Autodesk Fusion 360 part; units mm, degrees
sketch "Sketch2" plane through (0, 0, 0) normal (0, 1, 0) x (1, 0, 0)
  line L0 (0, 0) -> (42.015, 0)
  line L1 (42.015, 0) -> (42.015, -15.89)
  line L2 (42.015, -15.89) -> (0, -15.89)
  line L3 (0, -15.89) -> (0, 0)
  circle A0 centre (45.515, -7.945) radius 1.5
  line L4 (42.015, -7.945) -> (48.69, -7.945)
  spline S0 degree 5 poles (42.015, -12.945) (42.5156, -12.7419) (43.4745, -12.3366) (44.7863, -11.7309) (46.2763, -10.9278) (47.6689, -9.93) (48.5399, -8.9364) (48.8392, -7.945) (48.5399, -6.9536) (47.6689, -5.96) (46.2763, -4.9622) (44.7863, -4.1591) (43.4745, -3.5534) (42.5156, -3.1481) (42.015, -2.945) knots 0 0 0 0 0 0 0.1 0.2 0.3 0.4 0.5 0.6 0.7 0.8 0.9 1 1 1 1 1 1
  line L5 (20.92, -15.89) -> (20.92, 0)
  spline S1 degree 5 poles (-0.175, -12.945) (-0.6756, -12.7419) (-1.6345, -12.3366) (-2.9463, -11.7309) (-4.4363, -10.9278) (-5.8289, -9.93) (-6.6999, -8.9364) (-6.9992, -7.945) (-6.6999, -6.9536) (-5.8289, -5.96) (-4.4363, -4.9622) (-2.9463, -4.1591) (-1.6345, -3.5534) (-0.6756, -3.1481) (-0.175, -2.945) knots 0 0 0 0 0 0 0.1 0.2 0.3 0.4 0.5 0.6 0.7 0.8 0.9 1 1 1 1 1 1
  line L6 (40.2192, -13.6735) -> (43.8108, -12.2165)
  line L7 (43.8108, -3.6735) -> (40.2192, -2.2165)
  line L8 (1.6208, -13.6735) -> (-1.9708, -12.2165)
  line L9 (-1.9708, -3.6735) -> (1.6208, -2.2165)
  circle A1 centre (-3.675, -7.945) radius 1.5
  line L10 (-0.175, -7.945) -> (-6.85, -7.945)
  circle A2 centre (20.92, -9.45) radius 1
  circle A3 centre (20.92, -6.45) radius 1
  line L11 (-0.175, -12.945) -> (0, -13.016)
  line L12 (-0.175, -7.945) -> (0, -7.945)
  line L13 (-0.175, -2.945) -> (0, -2.874)
  dimension "d2" = 15.89
  dimension "d3" = 3
  dimension "d5" = 3.5
  dimension "d6" = 10
  dimension "d7" = 2.945
  dimension "d8" = 15.89
  dimension "d19" = 2
  dimension "d20" = 2
  dimension "d21" = 3
  dimension "d22" = 6.45
  dimension "d25" = 49.19
  dimension "d26" = 42.19
  dimension "d27" = 55.54
  dimension "d29" = 7.945
extrude "Extrude1" add sketch "Sketch2" along normal blind 6.35 contours L0 L2 L3 L5 A2 A3 | L0 L1 L2 L5 A2 A3 | L3 S1 L9 A1 L10 L12 L13 | L5 A3 | L5 A3 | L3 S1 L8 A1 L10 L11 L12 | L1 A0 L4 S0 | L1 A0 L4 S0 | L5 A2 | L5 A2
extrude "Extrude2" add sketch "Sketch2" against normal blind 3.56 contours L0 L2 L3 L5 A2 A3 | L0 L1 L2 L5 A2 A3 | L5 A3 | L5 A3 | L5 A2 | L5 A2
extrude "Extrude3" cut sketch "Sketch2" against normal blind 25 contours L5 A3 | L5 A3 | L5 A2 | L5 A2
equation "d5 = d4 - 1.5 mm - d3 / 2"
equation "d7 = ( d8 - d6 ) / 2"
equation "d12 = -9.91 mm + 6.35 mm"
equation "d29 = d2 / 2"
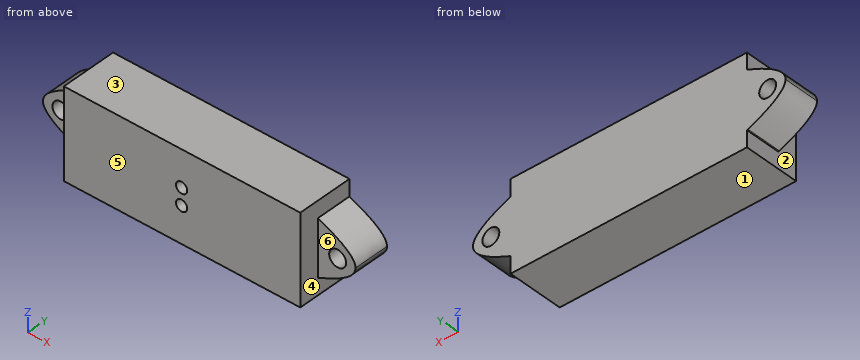
Check sheet for the modelled part. Datum: model origin and axes. Units: mm. Face numbers are marked on the shaded views. A direction names the side the tool comes from. Round coordinates to 2 decimals unless told otherwise and drop trailing zeros. Order: outer loops, then holes, each group sorted by start corner. A loop starts at its lowest first (then second) coordinate and runs counter-clockwise, first axis right, second up. Notation, with made-up numbers: (-29, 68.25) -> (6, 68.25) arc R27 cw to (6, 89.25) -> close; hole circle Ø5 at (73, -27.5). An arc over 180 degrees is marked (long way). Use CSV: the item, a comma, the result in double quotes.
(1) Cross-section at C-C (z = 1.5). Record the boundary of the cut face in (x, y) (3 decimals).
Worked out:
outline,"(0, -3.56) -> (42.015, -3.56) -> (42.015, 6.35) -> (0, 6.35) -> close"
(2) Cross-section at A-A (y = -2.5). Record the boundary of the cut face in (x, z) (3 decimals), and give its area (3 significant figures).
Worked out:
outline,"(0, 0) -> (42.015, 0) -> (42.015, 15.89) -> (0, 15.89) -> close; hole circle Ø2 at (20.92, 6.45); hole circle Ø2 at (20.92, 9.45)"
area,"661 mm²"
(3) Depth check by flat-ended pin: pin 1 (7.5 mm diameter, centred on x = 45.5, z = 8, fed in from -Y); pin 2 (0.6 mm diameter, centred on x = 20.5, z = 9.5, fed in from -Y); pin 3 (2.5 mm diameter, centred on x = -3.675, z = 7.945, fed in from -Y). Enter the tip coordinate at first touch or a pass-through.
Worked out:
pin 1,"y = -3.56"
pin 2,"y = 0"
pin 3,"through"
(4) Cross-section at D-D (y = 3.5). Count the separate pieces of the cut face and the enclosed holes in it, and give its area (3 significant figures).
Worked out:
separate pieces,"1"
enclosed holes,"2"
area,"742 mm²"
(5) Material ranges on line 1 along Z through (x, y) = (20.92, -1.95); line 2 along X through (y, z) = (-2.75, 9.45) (3 decimals); line 3 along X through (y, z) = (5.5, 7.5), recorded low to high. Write a range as from..to.
Worked out:
line 1,"0..5.45, 7.45..8.45, 10.45..15.89"
line 2,"0..19.92, 21.92..42.015"
line 3,"-6.79..-5.11, -2.24..44.08, 46.95..48.63"
(6) Cross-section at B-B (x = 20.92). Record the boundary of the cut face in (y, z).
Worked out:
outline,"(-3.56, 0) -> (6.35, 0) -> (6.35, 15.89) -> (-3.56, 15.89) -> (-3.56, 10.45) -> (0, 10.45) -> (0, 8.45) -> (-3.56, 8.45) -> (-3.56, 7.45) -> (0, 7.45) -> (0, 5.45) -> (-3.56, 5.45) -> close"
(7) Draft check along Z on the marked faces 1, 2 and 3. Enter one of: pulls with the +Z half, pulls with the -Z half, needs draft (parallel to the pull), parting line crosses it, or undercut.
Worked out:
face 1,"pulls with the -Z half"
face 2,"needs draft"
face 3,"pulls with the +Z half"
(8) Tool access check on the marked faces 4, 5 and 6. Record the directions out of +Z, -Z, +X, -X, +Y, -Y that give a thin tool (end or side, any length) a straight path to the whole face; none if there is none.
Worked out:
face 4,"+X, -Y"
face 5,"+Z, -Z, +X, -X, -Y"
face 6,"+Z, -Z, +X, -Y"
